```python
from build123d import *

# Parameters (mm, degrees)
F0_W     = 83.82
F0_H     = 10.16
F1_DEPTH = 193.04
F2_W     = 76.327
F2_H     = 185.547
F3_DEPTH = 10.16
F5_DEPTH = 25.4
F6_R     = 3.81
F7_R     = 4.8259


# Not quite as in the source:
# - a fillet or chamfer is up to 0.001 mm smaller than in the source, because OpenCascade refuses the exact size


with BuildPart() as f1:
    # F0 (on Front) → F1 (new body)
    with BuildSketch(Plane.XZ):
        Polygon((-7.4224442948, 6.35), (-7.4224442948, 0), (76.3975557052, 0), (76.3975557052, 1.9571799405), align=None)
        with Locations((34.4875557052, -5.08)):
            Rectangle(F0_W, F0_H)
    extrude(amount=F1_DEPTH)

    # F2 (on face) → F3 (cut)
    with BuildSketch(Plane(origin=(0, 0, -10.16), x_dir=(1, 0, 0), z_dir=(0, 0, -1))):
        with Locations((34.4875557052, 96.52)):
            Rectangle(F2_W, F2_H)
    extrude(amount=-F3_DEPTH, mode=Mode.SUBTRACT)

    # F4 (on face) → F5 (cut)
    with BuildSketch(Plane(origin=(0, 0, 0), x_dir=(1, 0, 0), z_dir=(0, 0, -1))):
        with BuildLine():
            ThreePointArc((23.6090351158, 172.2802219646), (28.189972413, 146.1460578684), (50.3625557052, 160.7185))
            ThreePointArc((50.3625557052, 160.7185), (49.0599978368, 167.0160832922), (45.3660762946, 172.2802219646))
            ThreePointArc((45.3660762946, 172.2802219646), (34.4875557052, 176.5935), (23.6090351158, 172.2802219646))
        make_face()
        with BuildLine():
            ThreePointArc((23.6090351158, 172.2802219646), (34.4875557052, 176.5935), (45.3660762946, 172.2802219646))
            Line((45.3660762946, 172.2802219646), (45.3660762946, 189.2935))
            Line((45.3660762946, 189.2935), (23.6090351158, 189.2935))
            Line((23.6090351158, 189.2935), (23.6090351158, 172.2802219646))
        make_face()
    extrude(amount=-F5_DEPTH, mode=Mode.SUBTRACT)

    # F6
    f6_edges = [f1.edges().sort_by_distance(p)[0] for p in [
        (59.008566, -189.2935, 0),
        (9.966545, -189.2935, 0),
        (-3.675944, -96.52, 0),
        (72.651056, -96.52, 0),
        (34.487556, -3.7465, 0),
    ]]
    fillet(f6_edges, radius=F6_R)

    # F7 (radius 4.826 in the source; OpenCascade refuses exactly that, so slightly less here)
    f7_edges = [f1.edges().sort_by_distance(p)[0] for p in [
        (45.366076, -189.2935, 1.791735),
        (23.609035, -189.2935, 2.361855),
    ]]
    fillet(f7_edges, radius=F7_R)


solid = f1.part
```
The model under review builds one solid part; all positions refer to its coordinate system, in mm. A direction names the side the tool comes from. Round coordinates to 2 decimals unless told otherwise and drop trailing zeros. Write each loop counter-clockwise with the first axis right and the second up, starting at its lowest first coordinate (ties: lowest second). Pieces come first, ordered by that corner, then holes. Notation, with made-up numbers: M 35.25,29.25 L 90.25,29.25 A35 cw 90.25,63.25 Z; hole C 18,2 d1. An arc over 180 degrees is marked long. Use CSV: the item, a comma, the result in double quotes. Start each with the question number.
(1) The part is to be moulded in two halves that separate along Y. For faces 4 (the face through (34, -193.04, -4)), 5 (the face through (35.074, -95.169, 4.123)), 6 (the face through (56.82, -188.21, -1.15)), 7 (the face through (34, -98, 0)), say which applies: +Y half, -Y half, draft (parallel to the pull), parting line (faces both ways), or undercut.
(2) We need section C-C, the plane x = 9. State the section outline as (y, z) points.
(3) Tool access review of faces 1 (the face through (45.366, -178, 2)), 2 (the face through (76.398, -95, -4)), 3 (the face through (71.565, -97.819, -1.146)): name each direction out of +Z, -Z, +X, -X, +Y, -Y from which nothing blocks a thin tool from reaching the whole face with its end or side.
(4) We need section B-B, the plane x = 42.5. State the section outline as (y, z) points.
(5) We need section A-A, the plane y = -86. State the section outline as (x, z) points.
(6) Clearance check with flat-ended pins moving along their axes: P1, Ø1.5, axis at x = 60, y = -127, coming from the +Z side; P2, Ø2, axis at x = 25, y = -70, coming from the +Z side; P3, Ø8, axis at x = 51.5, y = -40.5, coming from the -Z side. State where each tip first meets the part, or that it passes through.
(7) For line 1 along X through (y, z) = (-138, -8.25); line 2 along Y through (x, z) = (49.5, -5.5); line 3 along X through (y, z) = (-124.5, -1.5), list the stretches that pass through material, from the lowest coordinate up.
Findings:
1,face 4,"-Y half"
1,face 5,"draft"
1,face 6,"undercut"
1,face 7,"undercut"
2,outline,"M -193.04,-10.16 L -189.29,-10.16 L -189.29,-3.81 A3.81 cw -185.48,0 L -7.56,0 A3.81 cw -3.75,-3.81 L -3.75,-10.16 L 0,-10.16 L 0,5.49 L -193.04,5.49 Z"
3,face 1,"+Z, -Z"
3,face 2,"+Z, -Z, +X, +Y, -Y"
3,face 3,"-Z"
4,outline,"M -193.04,-10.16 L -189.29,-10.16 L -189.29,-3.81 A3.81 cw -188.88,-2.08 L -188.88,3.73 L -193.04,3.73 Z; M -147.01,0 L -7.56,0 A3.81 cw -3.75,-3.81 L -3.75,-10.16 L 0,-10.16 L 0,3.73 L -147.01,3.73 Z"
5,outline,"M -7.42,-10.16 L -3.68,-10.16 L -3.68,-3.81 A3.81 cw 0.13,0 L 68.84,0 A3.81 cw 72.65,-3.81 L 72.65,-10.16 L 76.4,-10.16 L 76.4,1.96 L -7.42,6.35 Z"
6,P1,"z = 2.86"
6,P2,"z = 4.7"
6,P3,"z = 0"
7,line 1,"-7.42 to -3.68, 72.65 to 76.4"
7,line 2,"-193.04 to -189.29, -3.75 to 0"
7,line 3,"-7.42 to -2.9, 71.87 to 76.4"
